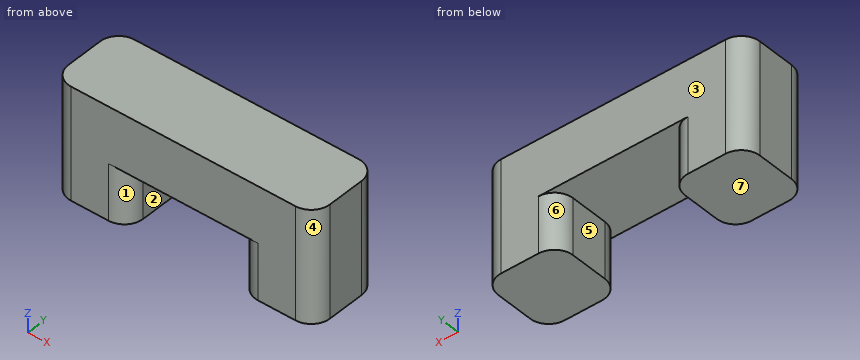
from build123d import *

# Parameters (mm, degrees)
F0_W     = 4
F0_H     = 4
F1_DEPTH = 3
F2_W     = 4
F2_H     = 4
F2_W_2   = 10
F3_DEPTH = 3
F4_R     = 1


with BuildPart() as f1:
    # F0 (on Top) → F1 (new body)
    with BuildSketch(Plane.XY):
        with Locations((-5, 0)):
            Rectangle(F0_W, F0_H)
        with Locations((5, 0)):
            Rectangle(F0_W, F0_H)
    extrude(amount=F1_DEPTH)

    # F2 (on face) → F3 (join)
    with BuildSketch(Plane.XY.offset(3)):
        with Locations((-5, 0)):
            Rectangle(F2_W, F2_H)
        with Locations((2, 0)):
            Rectangle(F2_W_2, F2_H)
    extrude(amount=F3_DEPTH)

    # F4
    f4_edges = [f1.edges().sort_by_distance(p)[0] for p in [
        (-7, -2, 3),
        (-3, -2, 1.5),
        (-3, 2, 1.5),
        (3, -2, 1.5),
        (7, -2, 3),
        (7, 2, 3),
        (3, 2, 1.5),
        (-7, 2, 3),
    ]]
    fillet(f4_edges, radius=F4_R)


solid = f1.part
The model under review builds one solid part; all positions refer to its coordinate system, in mm. Face numbers are marked on the shaded views. A direction names the side the tool comes from. Coordinates: 2 decimals unless noted, no trailing zeros. Write each loop counter-clockwise with the first axis right and the second up, starting at its lowest first coordinate (ties: lowest second). Pieces come first, ordered by that corner, then holes. Notation, with made-up numbers: (78.5, 55.5) -> (98.5, 55.5) arc R23 ccw to (98.5, 67.5) -> close; hole circle Ø7 at (52.25, -18). An arc over 180 degrees is marked (long way). Answer in a Markdown table with one row per item.
1. Wall thickness on probe 1 along X at (y, z) = (-0.85, 2.5); probe 2 along Z at (x, y) = (-1.25, -0.6); probe 3 along X at (y, z) = (1.6, 3.3): over which ranges is each line inside the solid? List them lowest first. Write a range as [from, to].
Answers below:
| item | result |
|---|---|
| probe 1 | x = [-7, -3], [3, 7] |
| probe 2 | z = [3, 6] |
| probe 3 | x = [-6.8, 6.8] |
2. We need section A-A, the plane z = 2.2. State the section outline as (x, y) points, and give its area (3 significant figures).
Answers below:
| item | result |
|---|---|
| outline | (-7, -1) arc R1 ccw to (-6, -2) -> (-4, -2) arc R1 ccw to (-3, -1) -> (-3, 1) arc R1 ccw to (-4, 2) -> (-6, 2) arc R1 ccw to (-7, 1) -> close; (3, -1) arc R1 ccw to (4, -2) -> (6, -2) arc R1 ccw to (7, -1) -> (7, 1) arc R1 ccw to (6, 2) -> (4, 2) arc R1 ccw to (3, 1) -> close |
| area | 30.3 mm^2 |
3. We need section D-D, the plane x = -1.25. State the section outline as (y, z) points, and give its area (3 significant figures).
Answers below:
| item | result |
|---|---|
| outline | (-2, 3) -> (2, 3) -> (2, 6) -> (-2, 6) -> close |
| area | 12.0 mm^2 |
4. Draft analysis for pull direction X (two halves, no side actions). For the marked faces 4, 5, 6 and 7, state which applies: +X half, -X half, draft (parallel to the pull), parting line (faces both ways), or undercut.
Answers below:
| item | result |
|---|---|
| face 4 | +X half |
| face 5 | undercut |
| face 6 | undercut |
| face 7 | draft |
5. We need section B-B, the plane y = -1.6. State the section outline as (x, z) points, and give its area (3 significant figures).
Answers below:
| item | result |
|---|---|
| outline | (-6.8, 0) -> (-3.2, 0) -> (-3.2, 3) -> (3.2, 3) -> (3.2, 0) -> (6.8, 0) -> (6.8, 6) -> (-6.8, 6) -> close |
| area | 62.4 mm^2 |
6. For the marked faces 1, 2 and 3, list the 3-axis set-ups (+Z, -Z, +X, -X, +Y, -Y) from which the entire face can be reached by the end or side of a thin tool; tool diameter is ignored.
Answers below:
| item | result |
|---|---|
| face 1 | -Z, -Y |
| face 2 | -Z, +Y, -Y |
| face 3 | +Z, -Z, +X, -X, +Y |
7. We need section C-C, the plane z = 5. State the section outline as (x, y) points.
Answers below:
| item | result |
|---|---|
| outline | (-7, -1) arc R1 ccw to (-6, -2) -> (6, -2) arc R1 ccw to (7, -1) -> (7, 1) arc R1 ccw to (6, 2) -> (-6, 2) arc R1 ccw to (-7, 1) -> close |
